Verification items for the finished model (mm, model axes). A direction names the side the tool comes from. Coordinates: 2 decimals unless noted, no trailing zeros. Write each loop counter-clockwise with the first axis right and the second up, starting at its lowest first coordinate (ties: lowest second). Pieces come first, ordered by that corner, then holes. Notation, with made-up numbers: (-30, 40) - (-21, 40) arc R19 cw to (-21, 55) - close; hole circle Ø5 at (79.25, 59.5). An arc over 180 degrees is marked (long way). Use one line per item in the form item = value. Start each with the question number.
(1) Gauge pin test, flat ends, axial feed: pin 1 Ø1 at (x, y) = (-3.5, 24.5) entering from -Z; pin 2 Ø1.2 at (y, z) = (-14.95, -67.05) entering from -X; pin 3 Ø4 at (x, z) = (-15.5, -63.5) entering from +Y. Record the tip position at first contact, or that the pin passes through.
(2) Sectioned sample at D-D (y = 15.5). Record the cut outline in (x, z), and give its area (3 significant figures).
(3) Tool access check on faces 4 (the flat face through (24, -6, -76)), 5 (the flat face through (0, 23, -22)), 6 (the cylindrical face through (-24, -17.6, -72.8)). Record the directions out of +Z, -Z, +X, -X, +Y, -Y that give a thin tool (end or side, any length) a straight path to the whole face; none if there is none.
(4) Sectioned sample at A-A (y = -17). Record the cut outline in (x, z), and give its area (3 significant figures).
(5) Mould release check, pull along Z, two halves, no side actions. Record for faces 1 (the flat face through (0, -24, -80)), 2 (the cylindrical face through (23.986, -4.126, -67.433)), 3 (the flat face through (0, -25, -39)): released by +Z, released by -Z, zero draft, split by the parting line, or undercut.
(6) Material ranges on line 1 (Y direction, x = -23.5, z = -72); line 2 (X direction, y = -2, z = -49.5), recorded low to high. Write a range as [from, to].
(7) Sectioned sample at B-B (x = -14). Record the cut outline in (y, z).
(8) Sectioned sample at C-C (z = -65). Record the cut outline in (x, y).
Autodesk Inventor part; units mm, degrees
ref_plane "YZ Plane" through (0, 0, 0) normal (1, 0, 0) x (0, 1, 0)
ref_plane "XZ Plane" through (0, 0, 0) normal (0, 1, 0) x (-1, 0, 0)
ref_plane "XY Plane" through (0, 0, 0) normal (0, 0, 1) x (1, 0, 0)
sketch "スケッチ1" plane through (0, 0, 0) normal (0, 0, 1) x (1, 0, 0)
  line L0 (-25, 25) -> (25, 25)
  line L1 (25, 25) -> (25, -25)
  line L2 (25, -25) -> (-25, -25)
  line L3 (-25, -25) -> (-25, 25)
  line L4 (-23, 23) -> (23, 23)
  line L5 (23, 23) -> (23, -23)
  line L6 (23, -23) -> (-23, -23)
  line L7 (-23, -23) -> (-23, 23)
  point P0 (0, 0)
  dimension "d0" = 50
  dimension "d2" = 50
  dimension "d3" = 46
  dimension "d4" = 23
  dimension "d5" = 23
  dimension "d6" = 25
  dimension "d7" = 46
  dimension "d8" = 25
extrude "押し出し1" add sketch "スケッチ1" against normal blind 80
sketch "スケッチ2" plane through (25, -25, 0) normal (1, 0, 0) x (0, 0, -1)
  line L0 (0, 0) -> (80, 0)
  line L1 (80, 50) -> (80, 0)
  line L2 (80, 19) -> (72, 19)
  line L3 (72, 11) -> (80, 11)
  line L4 (80, 11) -> (80, 19)
  arc A0 (72, 19) -> (72, 11) centre (72, 15) ccw
  point P0 (0, 25)
  dimension "d11" = 8
  dimension "d15" = 4
  dimension "d16" = 8
  dimension "d17" = 15
  dimension "d18" = 8
  dimension "d19" = 8
extrude "押し出し2" cut sketch "スケッチ2" against normal blind 60
sketch "スケッチ3" plane through (25, -25, 0) normal (1, 0, 0) x (0, 0, -1)
  arc A0 (72, 19) -> (72, 11) centre (72, 15) ccw
  circle A1 centre (72, 22) radius 1
  point P0 (0, 25)
  dimension "d22" = 0
  dimension "d23" = 7
  dimension "d24" = 2
hole "穴1" at (25, -3, -72) direction (-1, 0, 0) diameter 2 end through all
pattern_circular "円形状パターン1" count 5 over 180 about axis through (25, -10, -72) along (1, 0, 0) of "穴1"
sketch "スケッチ4" plane through (-25, 25, 0) normal (0, 1, 0) x (1, 0, 0)
  line L0 (50, 0) -> (50, 80)
  line L1 (0, 80) -> (50, 80)
  line L2 (2, 80) -> (48, 80)
  line L3 (48, 80) -> (48, 45)
  line L4 (48, 45) -> (2, 45)
  line L5 (2, 45) -> (2, 80)
  point P0 (25, 0)
  dimension "d35" = 46
  dimension "d37" = 2
  dimension "d38" = 35
extrude "押し出し3" cut sketch "スケッチ4" against normal blind 30
properties part number "Arm_Fifth_Flame"
Answers below:
q1.pin_1 = -45
q1.pin_2 = through
q1.pin_3 = -23
q2.outline = (-25, -80) - (-23, -80) - (-23, 0) - (-25, 0) - close; (23, -80) - (25, -80) - (25, 0) - (23, 0) - close
q2.area = 320 mm2
q3.face_4 = -Z, +X, -X
q3.face_5 = +Z, -Z
q3.face_6 = +X, -X
q4.outline = (-25, -80) - (-23, -80) - (-23, -73) - (-25, -73) - close; (-25, -71) - (-23, -71) - (-23, 0) - (-25, 0) - close; (23, -80) - (25, -80) - (25, -73) - (23, -73) - close; (23, -71) - (25, -71) - (25, 0) - (23, 0) - close
q4.area = 312 mm2
q5.face_1 = released by -Z
q5.face_2 = undercut
q5.face_3 = zero draft
q6.line_1 = [-25, -18], [-16, -14], [-6, -4], [-2, 25]
q6.line_2 = [-25, -23], [23, 25]
q7.outline = (-25, -80) - (-23, -80) - (-23, 0) - (-25, 0) - close; (23, -45) - (25, -45) - (25, 0) - (23, 0) - close
q8.outline = (-25, -25) - (25, -25) - (25, -11) - (23, -11) - (23, -23) - (-23, -23) - (-23, -11) - (-25, -11) - close; (-25, -9) - (-23, -9) - (-23, 25) - (-25, 25) - close; (23, -9) - (25, -9) - (25, 25) - (23, 25) - close
